For this review, take the finished solid that the model builds, in its own axes (mm). A direction names the side the tool comes from. Round coordinates to 2 decimals unless told otherwise and drop trailing zeros. Loops run counter-clockwise (first coordinate to the right, second up) from the corner with the lowest first, then second, coordinate; pieces in that order, holes last.
1) Tool access review of faces 5 (the flat face through (-2, -5, 4)), 6 (the flat face through (6, -5, -6)), 7 (the flat face through (6, -5, 6)): name each direction out of +Z, -Z, +X, -X, +Y, -Y from which nothing blocks a thin tool from reaching the whole face with its end or side.
2) Mouldability with a two-part tool opening along Z and no side actions: class faces 1 (the cylindrical face through (-6.69, -4.93, -2.87)), 2 (the flat face through (5, -5, -3)), 3 (the flat face through (0, 2, 10)), 4 (the cylindrical face through (-4.559, -4.93, -1.566)) as pulls with the +Z half, pulls with the -Z half, needs draft (parallel to the pull), parting line crosses it, or undercut.
3) Take a section at B-B (z = 4.5). State the section outline as (x, y) points.
4) Take a section at A-A (y = -2.25). State the section outline as (x, z) points, then the cut area to 3 significant figures.
5) Wall thickness on L1, parallel to X at y = -4.75, z = -0.5; L2, parallel to X at y = -0.75, z = -1.5; L3, parallel to Y at x = 6.25, z = 7: over which ranges is each line inside the solid? List them lowest first.
6) Insertion check: pin 1 (3 mm diameter, centred on y = -4.5, z = -3, fed in from +X); pin 2 (3 mm diameter, centred on x = 6, y = -4, fed in from -Z); pin 3 (1.2 mm diameter, centred on x = 6, y = -6.5, fed in from +Z). Each pin has a flat end and moves straight along its axis. Give the tip position at first contact, or say it passes through.
7) Take a section at D-D (x = 8.25). State the section outline as (y, z) points.
8) Take a section at C-C (x = 1.25). State the section outline as (y, z) points.
Autodesk Inventor part; units mm, degrees
ref_plane "YZ Plane" through (0, 0, 0) normal (1, 0, 0) x (0, 1, 0)
ref_plane "XZ Plane" through (0, 0, 0) normal (0, 1, 0) x (-1, 0, 0)
ref_plane "XY Plane" through (0, 0, 0) normal (0, 0, 1) x (1, 0, 0)
sketch "Sketch1" plane through (0, 0, 0) normal (0, 1, 0) x (-1, 0, 0)
  line L0 (-10, -10) -> (10, -10)
  line L1 (10, -10) -> (10, 10)
  line L2 (10, 10) -> (-10, 10)
  line L3 (-10, 10) -> (-10, -10)
  line L4 (-10, -10) -> (10, 10) construction
  line L5 (10, -10) -> (-10, 10) construction
  point P0 (0, 0)
  dimension "d0" = 20
  dimension "d1" = 20
extrude "Extrusion1" add sketch "Sketch1" along normal blind 5
sketch "Sketch2" plane through (0, 0, 0) normal (0, 1, 0) x (-1, 0, 0)
  arc A0 (-2.7434, -2.7839) -> (2, 5.5) centre (2, 0) ccw
  line L0 (2, 0) -> (-2.7434, -2.7839) construction
  line L1 (2, 0) -> (2, 5.5) construction
  arc A1 (-0.5873, -1.5185) -> (2, 3) centre (2, 0) ccw
  line L2 (2, 5.5) -> (2, 3)
  line L3 (-0.5873, -1.5185) -> (-5, 6)
  line L4 (-5, 6) -> (-7.5, 6)
  line L5 (-7.5, 6) -> (-7.5, -6)
  line L6 (-7.5, -6) -> (-5, -6)
  line L7 (-5, -6) -> (-5, 1.061)
  line L8 (-5, 1.061) -> (-2.7434, -2.7839)
  line L9 (-10, 10) -> (-10, -10)
  line L10 (7.5, 0) -> (7.5, -3.2169) construction
  line L11 (10, -10) -> (10, 10)
  line L12 (14, 0) -> (-14, 0)
  point P0 (0, 0)
  point P1 (2, 4.25)
  point P2 (-5, -2.4695)
  point P3 (-7.5, 0)
  dimension "d6" = 2.5
  dimension "d7" = 2.5
  dimension "d9" = 3
  dimension "d11" = 12
  dimension "d13" = 2.5
  dimension "d14" = 2.5
  dimension "d15" = 2.5
extrude "Extrusion2" add sketch "Sketch2" against normal blind 10 contours L8 L12 L3 A1 A0 | L12 A1 L2 A0 | L8 L7 L12 L5 L4 L3 | L7 L6 L5 L12
properties part number "2"
Response:
1. face 5: +Z, -Y
1. face 6: -Z, +X, -X, -Y
1. face 7: +Z, +X, -X, -Y
2. face 1: parting line crosses it
2. face 2: needs draft
2. face 3: pulls with the +Z half
2. face 4: undercut
3. outline: (-10, 0) - (-5.16, 0) - (-5.16, -10) - (-2, -10) - (-2, 0) - (4.12, 0) - (4.12, -10) - (7.5, -10) - (7.5, 0) - (10, 0) - (10, 5) - (-10, 5) - close
4. outline: (-2, 3) - (-2, 5.5) arc R5.5 ccw (long way) to (2.74, -2.78) - (5, 1.06) - (5, -6) - (7.5, -6) - (7.5, 6) - (5, 6) - (0.59, -1.52) arc R3 cw (long way) to start
4. area: 90.9 mm2
5. L1: x = -7.48 to -4.96, 1.19 to 4.08, 5 to 7.5
5. L2: x = -7.29 to -4.6, 0.6 to 3.5, 5 to 7.5
5. L3: y = 0 to 5
6. pin 1: stops at x = 7.5
6. pin 2: stops at z = -6
6. pin 3: stops at z = 6
7. outline: (0, -10) - (5, -10) - (5, 10) - (0, 10) - close
8. outline: (-10, -4.44) - (0, -4.44) - (0, -10) - (5, -10) - (5, 10) - (0, 10) - (0, -0.39) - (-10, -0.39) - close
